from build123d import *

# Parameters (mm, degrees)
ESBO_O1_W                     = 12
ESBO_O1_H                     = 16.75
RESSALTO_EXTRUS_O1_DEPTH      = 14.3
ESBO_O2_W                     = 15
ESBO_O2_H                     = 21
RESSALTO_EXTRUS_O2_DEPTH      = 2
ESBO_O3_W                     = 10
ESBO_O3_H                     = 15
CORTE_EXTRUS_O1_DEPTH         = 10
RESSALTO_EXTRUS_O3_DEPTH      = 4.7
RESSALTO_EXTRUS_O3_DEPTH_BACK = 4.7
FILETE1_R                     = 0.5
ESBO_O5_W                     = 8.5
ESBO_O5_H                     = 0.9
RESSALTO_EXTRUS_O4_DEPTH      = 7.1
CORTE_EXTRUS_O2_DEPTH         = 24.950891393
CORTE_EXTRUS_O2_DEPTH_BACK    = 24.950891393


with BuildPart() as part:
    # Esboço1 → Ressalto-extrusão1 (new body)
    with BuildSketch(Plane.XY):
        Rectangle(ESBO_O1_W, ESBO_O1_H)
    extrude(amount=RESSALTO_EXTRUS_O1_DEPTH)

    # Esboço2 → Ressalto-extrusão2 (add)
    with BuildSketch(Plane.XY.offset(14.3)):
        Rectangle(ESBO_O2_W, ESBO_O2_H)
    extrude(amount=RESSALTO_EXTRUS_O2_DEPTH)

    # Esboço3 → Corte-extrusão1 (cut)
    with BuildSketch(Plane.XY.offset(16.3)):
        Rectangle(ESBO_O3_W, ESBO_O3_H)
    extrude(amount=-CORTE_EXTRUS_O1_DEPTH, mode=Mode.SUBTRACT)

    # Esboço4 → Ressalto-extrusão3 (add, two sides: drawn at the far end of the back side and taken through both)
    with BuildSketch(Plane(origin=(0, 0, 0), x_dir=(0, 0, -1), z_dir=(1, 0, 0)).offset(-RESSALTO_EXTRUS_O3_DEPTH_BACK)):
        with BuildLine():
            ThreePointArc((-10.650515464, 7.488659794), (-12.165645544, -0.359367098), (-16.3, -7.2))
            ThreePointArc((-16.3, -7.2), (-18.509688847, -5.409688847), (-20.3, -3.2))
            ThreePointArc((-20.3, -3.2), (-17.43047856, 1.665568677), (-16.3, 7.2))
            ThreePointArc((-16.3, 7.2), (-13.490389917, 7.640488371), (-10.650515464, 7.488659794))
        make_face()
    extrude(amount=RESSALTO_EXTRUS_O3_DEPTH + RESSALTO_EXTRUS_O3_DEPTH_BACK)

    # Filete1
    filete1_edges = [part.edges().sort_by_distance(p)[0] for p in [
        (0, 7.2, 16.3),
        (0, -3.2, 20.3),
    ]]
    fillet(filete1_edges, radius=FILETE1_R)

    # Esboço5 → Ressalto-extrusão4 (add)
    with BuildSketch(Plane(origin=(0, 0, 0), x_dir=(-1, 0, 0), z_dir=(0, 0, -1))):
        Rectangle(ESBO_O5_W, ESBO_O5_H)
        with Locations((0, -7.5)):
            Rectangle(ESBO_O5_W, ESBO_O5_H)
        with Locations((0, 7.5)):
            Rectangle(ESBO_O5_W, ESBO_O5_H)
    extrude(amount=RESSALTO_EXTRUS_O4_DEPTH)

    # Esboço7 → Corte-extrusão2 (cut, two sides: drawn at the far end of the back side and taken through both)
    with BuildSketch(Plane(origin=(0, 0, 0), x_dir=(1, 0, 0), z_dir=(0, 1, 0)).offset(-CORTE_EXTRUS_O2_DEPTH_BACK)):
        with BuildLine():
            Line((2.5, 2), (4.25, 2))
            Line((4.25, 2), (4.25, 7.1))
            Line((4.25, 7.1), (0.1, 7.1))
            ThreePointArc((0.1, 7.1), (1.160660172, 6.660660172), (1.6, 5.6))
            Line((1.6, 5.6), (1.6, 3.5))
            ThreePointArc((1.6, 3.5), (1.746446609, 3.146446609), (2.1, 3))
            Line((2.1, 3), (2.5, 3))
            Line((2.5, 3), (2.5, 2))
        make_face()
        with BuildLine():
            Line((-4.25, 7.1), (-4.25, 2))
            Line((-4.25, 2), (-2.5, 2))
            Line((-2.5, 2), (-2.5, 3))
            Line((-2.5, 3), (-2.1, 3))
            ThreePointArc((-2.1, 3), (-1.746446609, 3.146446609), (-1.6, 3.5))
            Line((-1.6, 3.5), (-1.6, 5.6))
            ThreePointArc((-1.6, 5.6), (-1.160660172, 6.660660172), (-0.1, 7.1))
            Line((-0.1, 7.1), (-4.25, 7.1))
        make_face()
        with BuildLine():
            ThreePointArc((0.5, 6.5), (0.853553391, 6.353553391), (1, 6))
            Line((1, 6), (1, 4.5))
            ThreePointArc((1, 4.5), (0.853553391, 4.146446609), (0.5, 4))
            Line((0.5, 4), (-0.5, 4))
            ThreePointArc((-0.5, 4), (-0.853553391, 4.146446609), (-1, 4.5))
            Line((-1, 4.5), (-1, 6))
            ThreePointArc((-1, 6), (-0.853553391, 6.353553391), (-0.5, 6.5))
            Line((-0.5, 6.5), (0.5, 6.5))
        make_face()
    extrude(amount=CORTE_EXTRUS_O2_DEPTH + CORTE_EXTRUS_O2_DEPTH_BACK, mode=Mode.SUBTRACT)


solid = part.part
CAD build for the part. Positions are in the model's coordinates, mm. A direction names the side the tool comes from. Coordinates: 2 decimals unless noted, no trailing zeros. Write each loop counter-clockwise with the first axis right and the second up, starting at its lowest first coordinate (ties: lowest second). Pieces come first, ordered by that corner, then holes. Notation, with made-up numbers: (19.5, 37.5) - (38.5, 37.5) arc R6 cw to (38.5, 45.5) - close; hole circle Ø8 at (49, -39.75). An arc over 180 degrees is marked (long way). Use a Markdown table: item, result. Add a question column.
Item 1: Band-saw the part on D-D, the plane z = 17. Give the cut face in (x, y), and give its area (3 significant figures).
Item 2: Mould opens along X. For faces 5 (the face through (-1, 0, -5)), 6 (the face through (1.15, -7.51, -6.67)), 7 (the face through (0, -0.45, -2)), 8 (the face through (0, -7.5, -4)) say: pulls with the +X half, pulls with the -X half, needs draft (parallel to the pull), parting line crosses it, or undercut.
Item 3: Drill centre lines: L1, parallel to X at y = 2.5, z = 7.5; L2, parallel to Y at x = 0, z = 16.25; L3, parallel to Y at x = 3.5, z = 16. Where is each one in solid material? Low to high. Write a range as from..to.
Item 4: Band-saw the part on A-A, the plane y = 3. Give the cut face in (x, z).
Item 5: Flat gauge pins, fed straight in: pin 1 (2 mm diameter, centred on x = 0, z = -3, fed in from +Y); pin 2 (1 mm diameter, centred on x = 0, y = -7.5, fed in from +Z); pin 3 (10 mm diameter, centred on y = 5, z = -2.5, fed in from -X). Where does each tip first touch, or does it go through?
Item 6: 3-axis set-ups, long thin cutter, end or side, ignore diameter. For faces 1 (the face through (-7, 0, 16.3)), 2 (the face through (-2.5, -7.5, -2.5)), 3 (the face through (-7, 0, 14.3)), 4 (the face through (3, 0, -2)): which of +Z, -Z, +X, -X, +Y, -Y reach the whole face in a straight line?
Item 7: Band-saw the part on B-B, the plane z = 11.5. Give the cut face in (x, y) (3 decimals).
Item 8: Band-saw the part on C-C, the plane y = 5.25. Give the cut face in (x, z).
Numbers:
| question | item | result |
|---|---|---|
| 1 | outline | (-4.7, -6.71) - (4.7, -6.71) - (4.7, 2.93) - (-4.7, 2.93) - close |
| 1 | area | 90.6 mm2 |
| 2 | face 5 | undercut |
| 2 | face 6 | pulls with the +X half |
| 2 | face 7 | needs draft |
| 2 | face 8 | undercut |
| 3 | L1 | -6..-5, 5..6 |
| 3 | L2 | -10.5..-7.5, -7.14..7.06, 7.5..10.5 |
| 3 | L3 | -10.5..-7.5, -6.85..7.27, 7.5..10.5 |
| 4 | outline | (-7.5, 14.3) - (-6, 14.3) - (-6, 0) - (6, 0) - (6, 14.3) - (7.5, 14.3) - (7.5, 16.3) - (5, 16.3) - (5, 6.3) - (-5, 6.3) - (-5, 16.3) - (-7.5, 16.3) - close; (-4.7, 11.16) - (4.7, 11.16) - (4.7, 16.98) - (-4.7, 16.98) - close |
| 5 | pin 1 | y = 7.95 |
| 5 | pin 2 | z = 16.6 |
| 5 | pin 3 | x = -6 |
| 6 | face 1 | +Z |
| 6 | face 2 | -Z, -X, +Y, -Y |
| 6 | face 3 | -Z |
| 6 | face 4 | -Z, +X, +Y, -Y |
| 7 | outline | (-6, -8.375) - (6, -8.375) - (6, 8.375) - (-6, 8.375) - close; hole (-5, -7.5) - (5, -7.5) - (5, 7.5) - (4.7, 7.5) - (4.7, 1.644) - (-4.7, 1.644) - (-4.7, 7.5) - (-5, 7.5) - close |
| 8 | outline | (-7.5, 14.3) - (-6, 14.3) - (-6, 0) - (6, 0) - (6, 14.3) - (7.5, 14.3) - (7.5, 16.3) - (5, 16.3) - (5, 6.3) - (-5, 6.3) - (-5, 16.3) - (-7.5, 16.3) - close; (-4.7, 10.79) - (4.7, 10.79) - (4.7, 16.48) - (-4.7, 16.48) - close |
